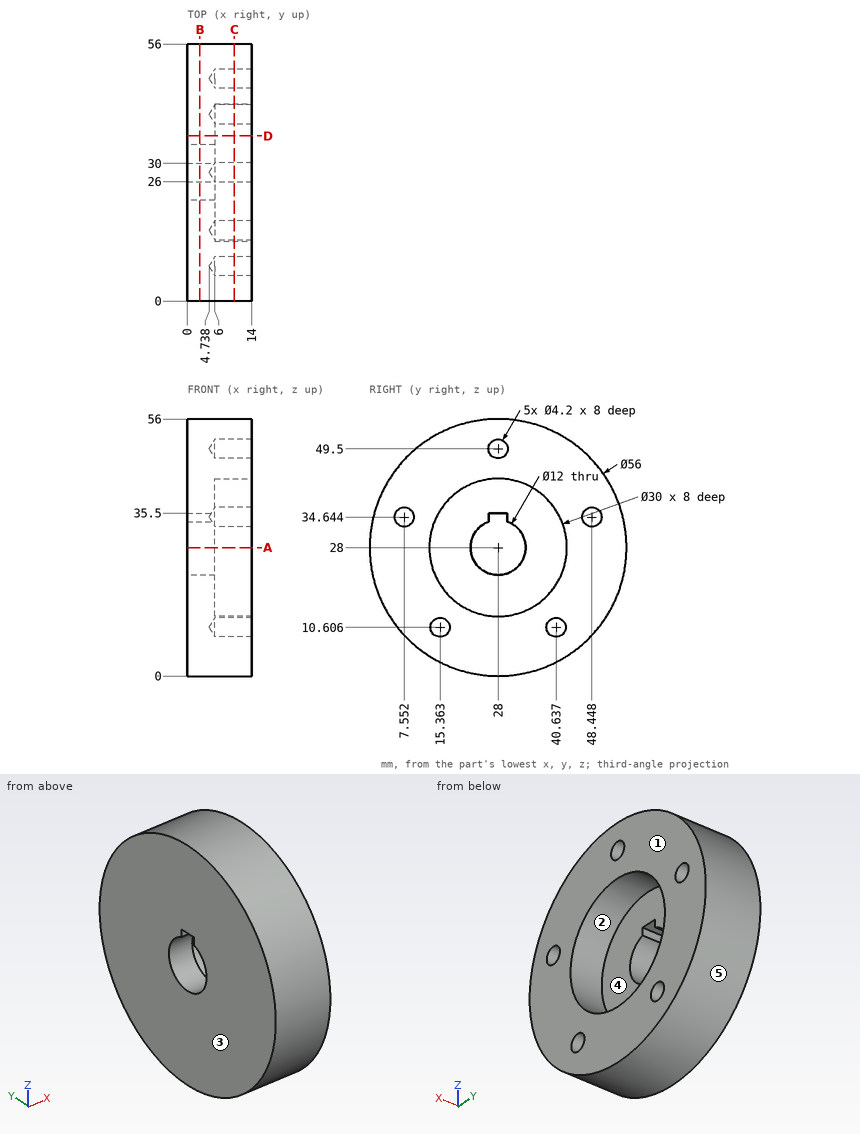
Geometry: see drawing. Coordinates: mm, zero at the bounding-box minimum. A direction names the side the tool comes from. Round coordinates to 2 decimals unless told otherwise and drop trailing zeros. Loops run counter-clockwise (first coordinate to the right, second up) from the corner with the lowest first, then second, coordinate; pieces in that order, holes last. Notation, with made-up numbers: (-8.5, 43.5) -> (16.5, 43.5) arc R13 cw to (16.5, 62.5) -> close; hole circle Ø3 at (-40, 52.5). An arc over 180 degrees is marked (long way). Write each question's results on one line, items separated by ' | '.
1. Section C-C (x = 10.25). Return loops of the section in (y, z).
Geometry results:
outline: circle Ø56 at (28, 28); hole circle Ø4.2 at (7.55, 34.64); hole circle Ø30 at (28, 28); hole circle Ø4.2 at (15.36, 10.61); hole circle Ø4.2 at (28, 49.5); hole circle Ø4.2 at (40.64, 10.61); hole circle Ø4.2 at (48.45, 34.64)
2. Ray query, line 1 (Z direction, x = 7.25, y = 15) (1 decimal); line 2 (Z direction, x = 8.5, y = 39); line 3 (X direction, y = 29.5, z = 21). Return the intervals inside material, ascending. Write a range as from..to.
Geometry results:
line 1: 3.2..8.5, 12.7..20.5, 35.5..52.8 | line 2: 2.25..9.29, 11.92..17.8, 38.2..53.75 | line 3: 0..6
3. Section D-D (y = 36). Return loops of the section in (x, z).
Geometry results:
outline: (0, 1.17) -> (14, 1.17) -> (14, 15.31) -> (6, 15.31) -> (6, 40.69) -> (14, 40.69) -> (14, 54.83) -> (0, 54.83) -> close
4. First-contact query: P1, Ø3, axis at x = 12, y = 30.5, coming from the -Z side; P2, Ø8, axis at x = 7, z = 25.5, coming from the +Y side; P3, Ø8, axis at x = 6, z = 43, coming from the -Y side; P4, Ø9.5, axis at y = 28, z = 28, coming from the -X side. Flat tips, straight axial feed; report the tip coordinate or a pass-through.
Geometry results:
P1: z = 0.02 | P2: y = 56 | P3: y = 2.25 | P4: through
5. Section A-A (z = 28). Return loops of the section in (x, y), and give its area (3 significant figures).
Geometry results:
outline: (0, 0) -> (14, 0) -> (14, 13) -> (6, 13) -> (6, 22) -> (0, 22) -> close; (0, 34) -> (6, 34) -> (6, 43) -> (14, 43) -> (14, 56) -> (0, 56) -> close | area: 472 mm2
6. Mould query, pull axis Z, two halves, no side actions, for the marked faces 3, 4 and 5. Classes: +Z half, -Z half, draft (parallel to the pull), parting line (faces both ways), or undercut.
Geometry results:
face 3: draft | face 4: undercut | face 5: parting line
7. Section B-B (x = 2.75). Return loops of the section in (y, z), and give its area (3 significant figures).
Geometry results:
outline: circle Ø56 at (28, 28); hole (26, 33.66) arc R6 ccw (long way) to (30, 33.66) -> (30, 35.5) -> (26, 35.5) -> close | area: 2,340 mm2
8. Set-up query: the marked faces 1 and 2. Return all of +Z, -Z, +X, -X, +Y, -Y with unobstructed straight access to the full face (end or side cutting, diameter ignored); none if empty.
Geometry results:
face 1: +Z, -Z, +X, +Y, -Y | face 2: +X
